Check sheet for the modelled part. Datum: model origin and axes. Units: mm. Give positions to 0.01 mm unless a question says otherwise; leave off trailing zeros. Order: outer loops, then holes, each group sorted by start corner. A loop starts at its lowest first (then second) coordinate and runs counter-clockwise, first axis right, second up. Notation, with made-up numbers: (-14, 75) - (20, 75) arc R24 ccw to (20, 109) - close; hole circle Ø8 at (-31.5, 25.25). An arc over 180 degrees is marked (long way). Answer in a Markdown table with one row per item.
from build123d import *

# Parameters (mm, degrees)
F0_W     = 25.4
F0_H     = 50.8
F1_DEPTH = 6.35
F3_D     = 5.1054
F3_DEPTH = 12.7
F3_TIP   = 1.5338169022
F4_R     = 14.3129
F5_DEPTH = 6.35


with BuildPart() as f1:
    # F0 (on Front) → F1 (new body)
    with BuildSketch(Plane.XZ):
        with Locations((-12.7, 0)):
            Rectangle(F0_W, F0_H)
        with BuildLine():
            Line((38.9980256121, 19.828853484), (0, 25.4))
            Line((0, 25.4), (0, -25.4))
            Line((0, -25.4), (38.9980256121, -19.828853484))
            ThreePointArc((38.9980256121, -19.828853484), (42.8971326142, -17.7032052569), (44.45, -13.5426741992))
            Line((44.45, -13.5426741992), (44.45, 0))
            Line((44.45, 0), (44.45, 13.5426741992))
            ThreePointArc((44.45, 13.5426741992), (42.8971326142, 17.7032052569), (38.9980256121, 19.828853484))
        make_face()
    extrude(amount=F1_DEPTH)

    # F3
    with Locations(Plane.XZ.offset(6.35)):
        with Locations((-12.7, 12.7), (-12.7, 0), (-12.7, -12.7)):
            Hole(F3_D / 2, depth=F3_DEPTH)
            with Locations((0, 0, -(F3_DEPTH + F3_TIP / 2))):  # 118° drill point
                Cone(0, F3_D / 2, F3_TIP, mode=Mode.SUBTRACT)

    # F4 (on face) → F5 (cut, through all)
    with BuildSketch(Plane.XZ.offset(6.35)):
        with Locations((25.4, 0)):
            Circle(F4_R)
    extrude(amount=-F5_DEPTH, mode=Mode.SUBTRACT)


solid = f1.part
(1) Cross-section at B-B, the plane x = -12.7. Record the cut outline in (y, z).
Geometry says:
| item | result |
|---|---|
| outline | (-6.35, -25.4) - (0, -25.4) - (0, -15.25) - (-6.35, -15.25) - close; (-6.35, -10.15) - (0, -10.15) - (0, -2.55) - (-6.35, -2.55) - close; (-6.35, 2.55) - (0, 2.55) - (0, 10.15) - (-6.35, 10.15) - close; (-6.35, 15.25) - (0, 15.25) - (0, 25.4) - (-6.35, 25.4) - close |
(2) Gauge pin test, flat ends, axial feed: P1, Ø1, axis at x = 14.5, y = -4.5, coming from the -Z side; P2, Ø3, axis at x = -11, z = -10.5, coming from the +Y side; P3, Ø1, axis at x = 25, y = -2.5, coming from the -Z side. Record the tip position at first contact, or that the pin passes through.
Geometry says:
| item | result |
|---|---|
| P1 | z = -23.4 |
| P2 | y = 0 |
| P3 | z = -21.9 |
(3) Cross-section at D-D, the plane x = 15.5. Record the cut outline in (y, z), then the cut area to 3 significant figures.
Geometry says:
| item | result |
|---|---|
| outline | (-6.35, -23.19) - (0, -23.19) - (0, -10.34) - (-6.35, -10.34) - close; (-6.35, 10.34) - (0, 10.34) - (0, 23.19) - (-6.35, 23.19) - close |
| area | 163 mm² |
(4) Cross-section at A-A, the plane z = 0. Record the cut outline in (x, y).
Geometry says:
| item | result |
|---|---|
| outline | (-25.4, -6.35) - (-15.25, -6.35) - (-15.25, 0) - (-25.4, 0) - close; (-10.15, -6.35) - (11.09, -6.35) - (11.09, 0) - (-10.15, 0) - close; (39.71, -6.35) - (44.45, -6.35) - (44.45, 0) - (39.71, 0) - close |
(5) Thickness scan on L1, parallel to X at y = -5.5, z = 0.5; L2, parallel to Z at x = -14.5, y = -0.75; L3, parallel to X at y = -2, z = 15. Record the ranges inside material, lowest first.
Geometry says:
| item | result |
|---|---|
| L1 | -25.4 to -15.2, -10.2 to 11.1, 39.7 to 44.45 |
| L2 | -25.4 to -14.51, -10.89 to -1.81, 1.81 to 10.89, 14.51 to 25.4 |
| L3 | -25.4 to -13.81, -11.59 to 44.28 |
(6) Cross-section at C-C, the plane y = -1.5. Record the cut outline in (x, z), then the cut area to 3 significant figures.
Geometry says:
| item | result |
|---|---|
| outline | (-25.4, -25.4) - (0, -25.4) - (39, -19.83) arc R6.35 ccw to (44.45, -13.54) - (44.45, 13.54) arc R6.35 ccw to (39, 19.83) - (0, 25.4) - (-25.4, 25.4) - close; hole circle Ø5.11 at (-12.7, -12.7); hole circle Ø5.11 at (-12.7, 0); hole circle Ø5.11 at (-12.7, 12.7); hole circle Ø28.63 at (25.4, 0) |
| area | 2,550 mm² |
(7) Mould release check, pull along X, two halves, no side actions. Record for faces 1 (the flat face through (-25.4, -3, 0)), 2 (the flat face through (-13, -3, 25.4)), 3 (the cylindrical face through (39.05, -3.22, 4.3)), 4 (the flat face through (19.226, -3.131, -22.653)): pulls with the +X half, pulls with the -X half, needs draft (parallel to the pull), parting line crosses it, or undercut.
Geometry says:
| item | result |
|---|---|
| face 1 | pulls with the -X half |
| face 2 | needs draft |
| face 3 | undercut |
| face 4 | pulls with the +X half |
